from build123d import *

# Parameters (mm, degrees)
F0_W     = 100
F0_H     = 100
F0_W_2   = 44
F0_H_2   = 44
F1_DEPTH = 20
F2_W     = 100
F2_H     = 100
F3_DEPTH = 5


with BuildPart() as f1:
    # F0 (on Front) → F1 (new body)
    with BuildSketch(Plane.XZ):
        with Locations((-4.064368, -0.652734)):
            Rectangle(F0_W, F0_H)
        with Locations((-28.064368, -24.652734)):
            Rectangle(F0_W_2, F0_H_2, mode=Mode.SUBTRACT)
        with Locations((19.935632, -24.652734)):
            Rectangle(F0_W_2, F0_H_2, mode=Mode.SUBTRACT)
        with Locations((-28.064368, 23.347266)):
            Rectangle(F0_W_2, F0_H_2, mode=Mode.SUBTRACT)
        with Locations((19.935632, 23.347266)):
            Rectangle(F0_W_2, F0_H_2, mode=Mode.SUBTRACT)
    extrude(amount=F1_DEPTH)

    # F2 (on face) → F3 (join)
    with BuildSketch(Plane(origin=(0, 0, 0), x_dir=(-1, 0, 0), z_dir=(0, 1, 0))):
        with Locations((4.064368, -0.652734)):
            Rectangle(F2_W, F2_H)
    extrude(amount=F3_DEPTH)


solid = f1.part
CAD build for the part. Positions are in the model's coordinates, mm. A direction names the side the tool comes from. Coordinates: 2 decimals unless noted, no trailing zeros. Loops run counter-clockwise (first coordinate to the right, second up) from the corner with the lowest first, then second, coordinate; pieces in that order, holes last. Notation, with made-up numbers: (-21, 29) -> (19, 29) arc R34 ccw to (19, 66) -> close; hole circle Ø7 at (4.25, 68.25). An arc over 180 degrees is marked (long way). One line per item, written item: value.
1. Drill centre lines: line 1 (X direction, y = -5.5, z = -16.5); line 2 (Z direction, x = -26, y = -12.75); line 3 (Y direction, x = 38, z = 31). Where is each one in solid material? Low to high. Write a range as [from, to].
Answers:
line 1: x = [-54.06, -50.06], [-6.06, -2.06], [41.94, 45.94]
line 2: z = [-50.65, -46.65], [-2.65, 1.35], [45.35, 49.35]
line 3: y = [0, 5]
2. Slice it at A-A on z = -5. Write the cut outline in (x, y).
Answers:
outline: (-54.06, -20) -> (-50.06, -20) -> (-50.06, 0) -> (-6.06, 0) -> (-6.06, -20) -> (-2.06, -20) -> (-2.06, 0) -> (41.94, 0) -> (41.94, -20) -> (45.94, -20) -> (45.94, 5) -> (-54.06, 5) -> close
3. Slice it at B-B on x = 37. Write the cut outline in (y, z), and give its area (3 significant figures).
Answers:
outline: (-20, -50.65) -> (5, -50.65) -> (5, 49.35) -> (-20, 49.35) -> (-20, 45.35) -> (0, 45.35) -> (0, 1.35) -> (-20, 1.35) -> (-20, -2.65) -> (0, -2.65) -> (0, -46.65) -> (-20, -46.65) -> close
area: 740 mm^2
4. Which spindle directions (+Z, -Z, +X, -X, +Y, -Y) get a long thin tool onto all of the face, cutting with end or side? Do faces 3 (the face through (41.936, -10, 23)), 4 (the face through (-3, -8, -50.653)). Say none if no direction does.
Answers:
face 3: -Y
face 4: -Z, +X, -X, +Y, -Y
5. Pull direction X, two halves, no side cores. Call faces 1 (the face through (-3, 5, 0)), 2 (the face through (20, 0, 24)): pulls with the +X half, pulls with the -X half, needs draft (parallel to the pull), parting line crosses it, or undercut.
Answers:
face 1: needs draft
face 2: undercut
6. Flat gauge pin, fed straight in: P1, Ø2, axis at x = -33, z = 33, coming from the -Y side. Where does the tip first touch, or does it go through?
Answers:
P1: stops at y = 0
7. Slice it at C-C on y = -15.25. Write the cut outline in (x, z), and give its area (3 significant figures).
Answers:
outline: (-54.06, -50.65) -> (45.94, -50.65) -> (45.94, 49.35) -> (-54.06, 49.35) -> close; hole (-50.06, -46.65) -> (-6.06, -46.65) -> (-6.06, -2.65) -> (-50.06, -2.65) -> close; hole (-50.06, 1.35) -> (-6.06, 1.35) -> (-6.06, 45.35) -> (-50.06, 45.35) -> close; hole (-2.06, -46.65) -> (41.94, -46.65) -> (41.94, -2.65) -> (-2.06, -2.65) -> close; hole (-2.06, 1.35) -> (41.94, 1.35) -> (41.94, 45.35) -> (-2.06, 45.35) -> close
area: 2,260 mm^2
